from build123d import *

# Parameters (mm, degrees)
SKETCH1_W           = 25.4
SKETCH1_H           = 25.4
SKETCH1_W_2         = 19.05
SKETCH1_H_2         = 19.05
BOSS_EXTRUDE1_DEPTH = 304.8
SKETCH2_R           = 2.413
CUT_EXTRUDE1_DEPTH  = 25.4


with BuildPart() as part:
    # Sketch1 → Boss-Extrude1 (new body)
    with BuildSketch(Plane(origin=(0, 0, 0), x_dir=(1, 0, 0), z_dir=(0, 1, 0))):
        Rectangle(SKETCH1_W, SKETCH1_H)
        Rectangle(SKETCH1_W_2, SKETCH1_H_2, mode=Mode.SUBTRACT)
    extrude(amount=BOSS_EXTRUDE1_DEPTH)

    # Sketch2 → Cut-Extrude1 (cut)
    with BuildSketch(Plane(origin=(12.7, 0, 0), x_dir=(0, 0, -1), z_dir=(1, 0, 0))):
        with Locations((0, 292.1)):
            Circle(SKETCH2_R)
        with Locations((0, 273.05)):
            Circle(SKETCH2_R)
        with Locations((0, 254)):
            Circle(SKETCH2_R)
        with Locations((0, 234.95)):
            Circle(SKETCH2_R)
        Polygon((-12.7, 0), (12.7, 11.844214517), (12.7, 0), align=None)
    extrude(amount=-CUT_EXTRUDE1_DEPTH, mode=Mode.SUBTRACT)


solid = part.part
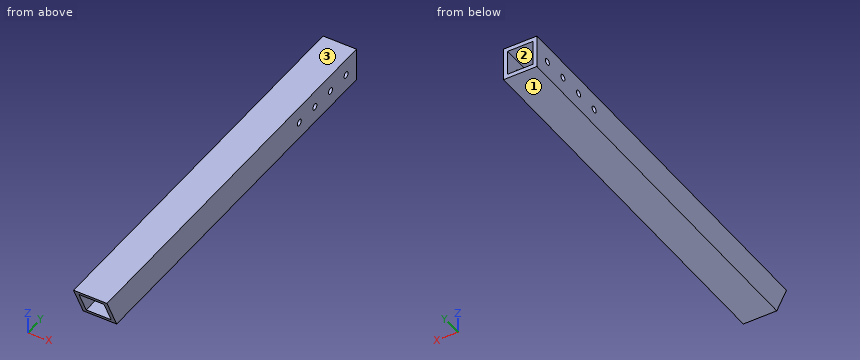
Here's how the part is built. I have some questions about the finished solid (model axes, mm). Face numbers are marked on the shaded views. Give positions to 0.01 mm unless a question says otherwise; leave off trailing zeros. Order: outer loops, then holes, each group sorted by start corner. A loop starts at its lowest first (then second) coordinate and runs counter-clockwise, first axis right, second up. Notation, with made-up numbers: (44, 48.25) -> (48, 48.25) arc R25 cw to (48, 67.25) -> close; hole circle Ø1 at (42.5, 42). An arc over 180 degrees is marked (long way). Use a Markdown table: item, result. Add a question column.
Item 1: If we mould it in two halves opening along Z, with no side actions, what happens to the marked faces 1, 2 and 3? For each: pulls with the +Z half, pulls with the -Z half, needs draft (parallel to the pull), parting line crosses it, or undercut.
Item 2: I need wall thicknesses on line 1 (X direction, y = 124.5, z = 3) (3 decimals); line 2 (Y direction, x = -11.1, z = 0). Which ranges of each line are inside material? Lowest first, please.
Item 3: Imagine slicing it at B-B on y = 38. Please give me the cut outline in (x, z) (3 decimals).
Item 4: Imagine slicing it at C-C on z = -6.25. Please give me the cut outline in (x, y) (3 decimals).
Item 5: Imagine slicing it at A-A on x = -3.5. Please give me the cut outline in (y, z) (3 decimals), plus the area to 3 significant figures.
Item 6: Will this pin go through, and if not, where does the flat tip stop? pin 1 (10 mm diameter, centred on x = -7.5, z = 1, fed in from +Y).
Data:
| question | item | result |
|---|---|---|
| 1 | face 1 | pulls with the -Z half |
| 1 | face 2 | undercut |
| 1 | face 3 | pulls with the +Z half |
| 2 | line 1 | x = -12.7 to -9.525, 9.525 to 12.7 |
| 2 | line 2 | y = 5.92 to 232.54, 237.36 to 251.59, 256.41 to 270.64, 275.46 to 289.69, 294.51 to 304.8 |
| 3 | outline | (-12.7, -12.7) -> (12.7, -12.7) -> (12.7, 12.7) -> (-12.7, 12.7) -> close; hole (-9.525, -9.525) -> (9.525, -9.525) -> (9.525, 9.525) -> (-9.525, 9.525) -> close |
| 4 | outline | (-12.7, 8.837) -> (-9.525, 8.837) -> (-9.525, 304.8) -> (-12.7, 304.8) -> close; (9.525, 8.837) -> (12.7, 8.837) -> (12.7, 304.8) -> (9.525, 304.8) -> close |
| 5 | outline | (0, 12.7) -> (1.481, 9.525) -> (304.8, 9.525) -> (304.8, 12.7) -> close; (10.364, -9.525) -> (11.844, -12.7) -> (304.8, -12.7) -> (304.8, -9.525) -> close |
| 5 | area | 1,900 mm² |
| 6 | pin 1 | stops at y = 304.8 |
